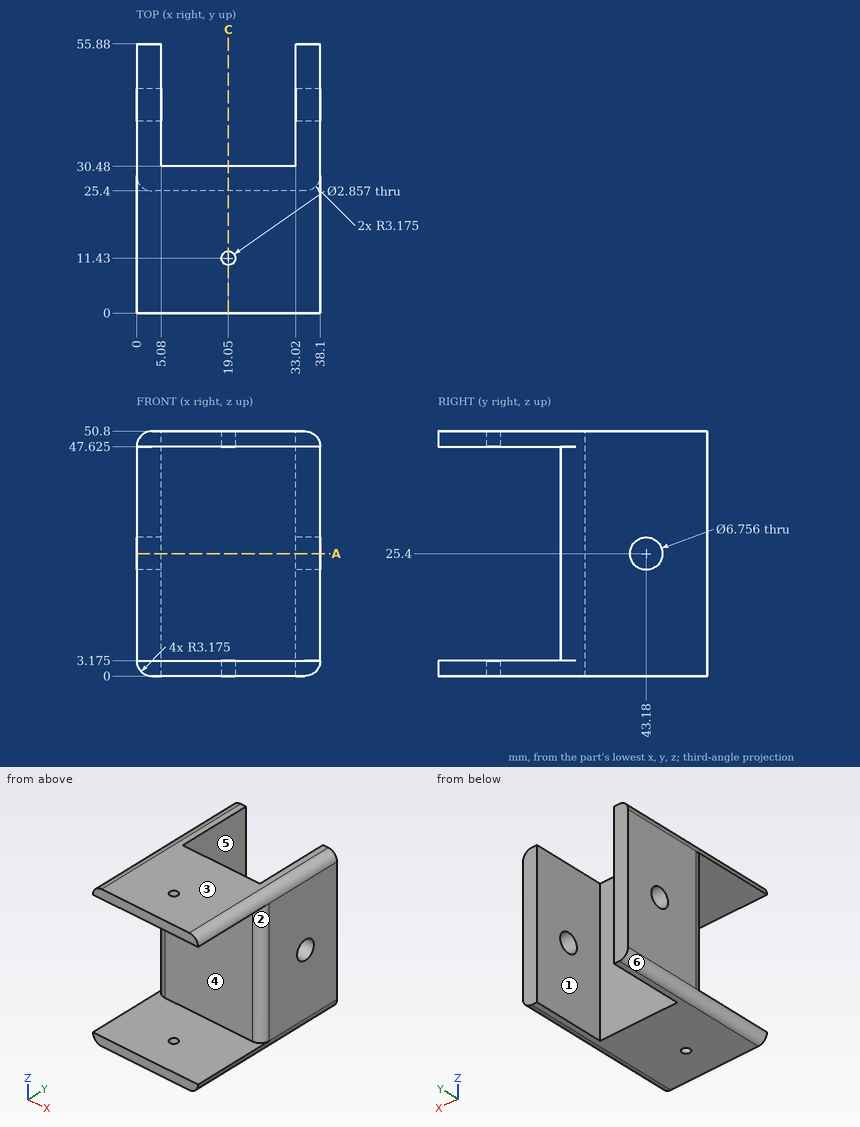
Verification items for this drawing (mm, ordinates from the low corner). A direction names the side the tool comes from. Coordinates: 2 decimals unless noted, no trailing zeros. Write each loop counter-clockwise with the first axis right and the second up, starting at its lowest first coordinate (ties: lowest second). Pieces come first, ordered by that corner, then holes. Notation, with made-up numbers: M 2,46.25 L 53,46.25 A28 cw 53,81.25 Z; hole C 62,28.5 d2. An arc over 180 degrees is marked long. Answer as a JSON object with one key per item and string values. Group by question number.
(1) Tool access check on the marked faces 1, 2 and 3. Record the directions out of +Z, -Z, +X, -X, +Y, -Y that give a thin tool (end or side, any length) a straight path to the whole face; none if there is none.
(2) Cross-section at C-C, the plane x = 19.05. Record the cut outline in (y, z) (1 decimal), and give its area (3 significant figures).
(3) Cross-section at A-A, the plane z = 25.4. State how many separate pieces and enclosed holes the cut face has.
(4) Release check for a two-part mould opening along X. For the marked faces 4, 5 and 6 record: +X half, -X half, draft (parallel to the pull), parting line (faces both ways), or undercut.
(5) Gauge pin test, flat end, axial feed: pin 1 (5 mm diameter, centred on x = 18, z = 34.5, fed in from -Y). Record the tip position at first contact, or that the pin passes through.
(6) Material ranges on line 1 (X direction, y = 42, z = 36.5); line 2 (Z direction, x = 13, y = 23.5) (1 decimal); line 3 (Y direction, x = 19, z = 2), recorded low to high.
Reply:
{
 "1": {"face 1": "+Z, -Z, +Y", "face 2": "+X, -Y", "face 3": "+Z, +X, -X, +Y, -Y"},
 "2": {"outline": "M 0,0 L 10,0 L 10,3.2 L 0,3.2 Z; M 0,47.6 L 10,47.6 L 10,50.8 L 0,50.8 Z; M 12.9,0 L 30.5,0 L 30.5,50.8 L 12.9,50.8 L 12.9,47.6 L 25.4,47.6 L 25.4,3.2 L 12.9,3.2 Z", "area": "401 mm²"},
 "3": {"separate pieces": "3", "enclosed holes": "0"},
 "4": {"face 4": "draft", "face 5": "undercut", "face 6": "-X half"},
 "5": {"pin 1": "y = 25.4"},
 "6": {"line 1": "0 to 5.08, 33.02 to 38.1", "line 2": "0 to 3.2, 47.6 to 50.8", "line 3": "0 to 10, 12.86 to 30.48"}
}
